```python
from build123d import *

# Parameters (mm, degrees)
BOSS_EXTRUDE1_DEPTH = 13.97
SKETCH2_R           = 2.667
CUT_EXTRUDE1_DEPTH  = 13.97
SKETCH3_R           = 3.81
CUT_EXTRUDE2_DEPTH  = 4.826
SKETCH4_R           = 2.1082
CUT_EXTRUDE3_DEPTH  = 17.272
CHAMFER1_SIZE       = 0.762


with BuildPart() as part:
    # Sketch1 → Boss-Extrude1 (new body)
    with BuildSketch(Plane(origin=(0, 0, 0), x_dir=(1, 0, 0), z_dir=(0, 1, 0))):
        with BuildLine():
            Line((10.16, 14.9225), (0.381, 14.9225))
            Line((0.381, 14.9225), (0.381, 6.020456399))
            ThreePointArc((0.381, 6.020456399), (0, -6.0325), (-0.381, 6.020456399))
            Line((-0.381, 6.020456399), (-0.381, 14.9225))
            Line((-0.381, 14.9225), (-10.16, 14.9225))
            Line((-10.16, 14.9225), (-10.16, -16.8275))
            Line((-10.16, -16.8275), (-20.32, -16.8275))
            Line((-20.32, -16.8275), (-20.32, -23.1775))
            Line((-20.32, -23.1775), (20.32, -23.1775))
            Line((20.32, -23.1775), (20.32, -16.8275))
            Line((20.32, -16.8275), (10.16, -16.8275))
            Line((10.16, -16.8275), (10.16, 14.9225))
        make_face()
    extrude(amount=BOSS_EXTRUDE1_DEPTH)

    # Sketch2 → Cut-Extrude1 (cut)
    with BuildSketch(Plane(origin=(0, 0, 16.8275), x_dir=(-1, 0, 0), z_dir=(0, 0, -1))):
        with Locations((-15.24, 6.985)):
            Circle(SKETCH2_R)
        with Locations((15.24, 6.985)):
            Circle(SKETCH2_R)
    extrude(amount=-CUT_EXTRUDE1_DEPTH, mode=Mode.SUBTRACT)

    # Sketch3 → Cut-Extrude2 (cut)
    with BuildSketch(Plane.ZY.offset(10.16)):
        with Locations((-9.8425, 6.985)):
            Circle(SKETCH3_R)
    extrude(amount=-CUT_EXTRUDE2_DEPTH, mode=Mode.SUBTRACT)

    # Sketch4 → Cut-Extrude3 (cut)
    with BuildSketch(Plane.ZY.offset(5.334)):
        with Locations((-9.8425, 6.985)):
            Circle(SKETCH4_R)
    extrude(amount=-CUT_EXTRUDE3_DEPTH, mode=Mode.SUBTRACT)

    # Chamfer1
    chamfer1_edges = [part.edges().sort_by_distance(p)[0] for p in [
        (0, 0, 6.0325),
        (0, 13.97, 6.0325),
        (17.907, 6.985, 16.8275),
        (-12.573, 6.985, 16.8275),
        (-10.16, 6.985, -13.6525),
    ]]
    chamfer(chamfer1_edges, length=CHAMFER1_SIZE)


solid = part.part
```
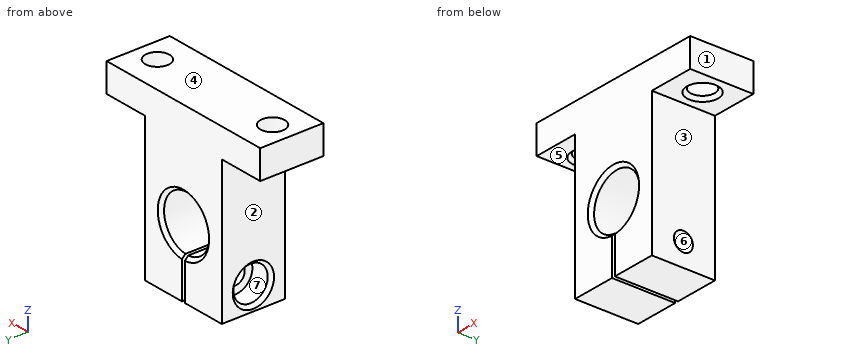
Geometry check sheet. Reference: the model listing, model coordinates, mm. Face numbers are marked on the shaded views. A direction names the side the tool comes from. Coordinates: 2 decimals unless noted, no trailing zeros. Order: outer loops, then holes, each group sorted by start corner. A loop starts at its lowest first (then second) coordinate and runs counter-clockwise, first axis right, second up. Notation, with made-up numbers: (-34, 40) - (3, 40) arc R29 ccw to (3, 74) - close; hole circle Ø11 at (73, 57). An arc over 180 degrees is marked (long way). Use one line per item in the form item = value.
1. Section check C-C (y = 12.5). Record the boundary of the cut face in (x, z) (1 decimal).
Here are the results:
outline = (-20.3, 16.8) - (-10.2, 16.8) - (-10.2, -14.9) - (-0.4, -14.9) - (-0.4, -6) arc R6 cw (long way) to (0.4, -6) - (0.4, -14.9) - (10.2, -14.9) - (10.2, 16.8) - (20.3, 16.8) - (20.3, 23.2) - (-20.3, 23.2) - close
2. Section check B-B (z = 0). Record the boundary of the cut face in (x, y).
Here are the results:
outline = (-10.16, 0) - (-6.79, 0) - (-6.03, 0.76) - (-6.03, 13.21) - (-6.79, 13.97) - (-10.16, 13.97) - close; (6.03, 0.76) - (6.79, 0) - (10.16, 0) - (10.16, 13.97) - (6.79, 13.97) - (6.03, 13.21) - close
3. Draft check along Z on the marked faces 4, 5, 6 and 7. Enter one of: pulls with the +Z half, pulls with the -Z half, needs draft (parallel to the pull), parting line crosses it, or undercut.
Here are the results:
face_4 = pulls with the +Z half
face_5 = pulls with the -Z half
face_6 = undercut
face_7 = undercut
4. Gauge pin test, flat ends, axial feed: pin 1 (4 mm diameter, centred on y = 7, z = -1.5, fed in from +X); pin 2 (2.5 mm diameter, centred on y = 8.5, z = -9, fed in from -X); pin 3 (3 mm diameter, centred on x = -16.5, y = 8, fed in from -Z). Record the tip position at first contact, or that the pin passes through.
Here are the results:
pin_1 = 10.16
pin_2 = -5.33
pin_3 = 17.14
5. Access from +Z, -Z, +X, -X, +Y, -Y to the whole of each face (thin tool, end or side, straight path). Record for the marked faces 1, 2 and 3.
Here are the results:
face_1 = +Z, -Z, +X, +Y, -Y
face_2 = -Z, -X, +Y, -Y
face_3 = -Z, +X, +Y, -Y
6. Scan lines: line 1 (X direction, y = 7.75, z = 0); line 2 (X direction, y = 2, z = -7.5); line 3 (Y direction, x = 15.24, z = 19.1). Record each from-to range of solid material in increasing order.
Here are the results:
line_1 = -10.16 to -6.03, 6.03 to 10.16
line_2 = -10.16 to -0.38, 0.38 to 10.16
line_3 = 0 to 4.32, 9.65 to 13.97
7. Section check D-D (z = 20). Record the boundary of the cut face in (x, y) (3 decimals), then the cut area to 3 significant figures.
Here are the results:
outline = (-20.32, 0) - (20.32, 0) - (20.32, 13.97) - (-20.32, 13.97) - close; hole circle Ø5.334 at (-15.24, 6.985); hole circle Ø5.334 at (15.24, 6.985)
area = 523 mm²
8. Section check A-A (x = 15.24). Record the boundary of the cut face in (y, z), then the cut area to 3 significant figures.
Here are the results:
outline = (0, 16.83) - (3.56, 16.83) - (4.32, 17.59) - (4.32, 23.18) - (0, 23.18) - close; (9.65, 17.59) - (10.41, 16.83) - (13.97, 16.83) - (13.97, 23.18) - (9.65, 23.18) - close
area = 54.3 mm²
